Design review of the part built by this model. Coordinates are the model's own, in mm. A direction names the side the tool comes from. Round coordinates to 2 decimals unless told otherwise and drop trailing zeros. Write each loop counter-clockwise with the first axis right and the second up, starting at its lowest first coordinate (ties: lowest second). Pieces come first, ordered by that corner, then holes. Notation, with made-up numbers: M -1.75,-39 L 42.25,-39 A4 cw 42.25,-32 Z; hole C 16.5,29.25 d6. An arc over 180 degrees is marked long. One line per question, with ' | ' between items. Start each with the question number.
Item 1: Insertion check: pin 1 Ø5 at (x, z) = (99.02, 0) entering from -Y; pin 2 Ø5 at (x, z) = (27.98, 0) entering from +Y; pin 3 Ø8 at (x, y) = (101.5, -17.5) entering from -Z. Each pin has a flat end and moves straight along its axis. Give the tip position at first contact, or say it passes through.
Item 2: Machinability: for faces 1 (the face through (63, -25.4, 5)), 2 (the face through (95.917, -28.531, -0.688)), 3 (the face through (127, 3, 0)), 4 (the face through (57.3, 28.62, -1.38)), 5 (the face through (63, 31.75, -11)), which of the approach directions +Z, -Z, +X, -X, +Y, -Y give a long, thin tool a straight path to every point of the face, cutting with its end or side? Answer none if there is none.
Item 3: Draft analysis for pull direction Z (two halves, no side actions). For faces 6 (the face through (24.955, -28.531, 0.954)), 7 (the face through (58, 26, 25.4)), 8 (the face through (58, 26, -25.4)), state which applies: released by +Z, released by -Z, zero draft, split by the parting line, or undercut.
Item 4: Add section B-B, the plane x = 63.5. State the section outline as (y, z) points (3 decimals), and give its area (3 significant figures).
Item 5: Add section A-A, the plane z = 0. State the section outline as (x, y) points (3 decimals).
Item 6: Add section C-C, the plane y = 10. State the section outline as (x, z) points.
Item 7: For L1, parallel to Y at x = 112, z = 4.5; L2, parallel to X at y = 35.5, z = 10, list the stretches that pass through material, from the lowest coordinate up.
Item 8: Add section D-D, the plane z = -12.5. State the section outline as (x, y) points.
```python
from build123d import *

# Parameters (mm, degrees)
SKETCH1_W               = 50.8
SKETCH1_H               = 63.5
BOSS_EXTRUDE1_DEPTH     = 127
SKETCH2_W               = 6.35
SKETCH2_H               = 50.8
BOSS_EXTRUDE2_DEPTH     = 6.35
CUT_EXTRUDE2_DEPTH      = 136.002851822
CUT_EXTRUDE2_DEPTH_BACK = 136.002851822
SKETCH4_W               = 114.3
SKETCH4_H               = 50.8
CUT_EXTRUDE3_REACH      = 146.244
SKETCH5_R               = 6.35
CUT_EXTRUDE4_REACH      = 146.244
SKETCH6_R               = 3.175


with BuildPart() as part:
    # Sketch1 → Boss-Extrude1 (new body)
    with BuildSketch(Plane(origin=(0, 0, 0), x_dir=(0, 0, -1), z_dir=(1, 0, 0))):
        Rectangle(SKETCH1_W, SKETCH1_H)
    extrude(amount=BOSS_EXTRUDE1_DEPTH)

    # Sketch2 → Boss-Extrude2 (add)
    with BuildSketch(Plane(origin=(0, 31.75, 0), x_dir=(1, 0, 0), z_dir=(0, 1, 0))):
        with Locations((123.825, 0)):
            Rectangle(SKETCH2_W, SKETCH2_H)
        with Locations((3.175, 0)):
            Rectangle(SKETCH2_W, SKETCH2_H)
    extrude(amount=BOSS_EXTRUDE2_DEPTH)

    # Sketch4 → Cut-Extrude2 (cut, two sides: drawn at the far end of the back side and taken through both)
    with BuildSketch(Plane.XY.offset(-CUT_EXTRUDE2_DEPTH_BACK)):
        with Locations((63.5, 0)):
            Rectangle(SKETCH4_W, SKETCH4_H)
    extrude(amount=CUT_EXTRUDE2_DEPTH + CUT_EXTRUDE2_DEPTH_BACK, mode=Mode.SUBTRACT)

    # Sketch5 → Cut-Extrude3 (cut, up to next)
    with BuildSketch(Plane(origin=(0, 31.75, 0), x_dir=(1, 0, 0), z_dir=(0, 1, 0)), mode=Mode.PRIVATE) as cut_extrude3_sk1:
        with Locations(Location((63.5, 0, 0), (0, 0, 270))):
            Circle(SKETCH5_R)
    cut_extrude3_tool1 = extrude(cut_extrude3_sk1.sketch, amount=-CUT_EXTRUDE3_REACH, mode=Mode.PRIVATE) & part.part
    add(cut_extrude3_tool1.solids().sort_by_distance((63.5, 31.75, 0))[0], mode=Mode.SUBTRACT)

    # Sketch6 → Cut-Extrude4 (cut, up to next)
    with BuildSketch(Plane(origin=(0, -25.4, 0), x_dir=(1, 0, 0), z_dir=(0, 1, 0)), mode=Mode.PRIVATE) as cut_extrude4_sk1:
        with Locations(Location((63.5, 0, 0), (0, 0, 180))):
            Circle(SKETCH6_R)
    cut_extrude4_tool1 = extrude(cut_extrude4_sk1.sketch, amount=-CUT_EXTRUDE4_REACH, mode=Mode.PRIVATE) & part.part
    # Sketch6 → Cut-Extrude4 (cut, up to next)
    with BuildSketch(Plane(origin=(0, -25.4, 0), x_dir=(1, 0, 0), z_dir=(0, 1, 0)), mode=Mode.PRIVATE) as cut_extrude4_sk2:
        with Locations(Location((27.983351472, 0, 0), (0, 0, 180))):
            Circle(SKETCH6_R)
    cut_extrude4_tool2 = extrude(cut_extrude4_sk2.sketch, amount=-CUT_EXTRUDE4_REACH, mode=Mode.PRIVATE) & part.part
    # Sketch6 → Cut-Extrude4 (cut, up to next)
    with BuildSketch(Plane(origin=(0, -25.4, 0), x_dir=(1, 0, 0), z_dir=(0, 1, 0)), mode=Mode.PRIVATE) as cut_extrude4_sk3:
        with Locations(Location((99.016648528, 0, 0), (0, 0, 270))):
            Circle(SKETCH6_R)
    cut_extrude4_tool3 = extrude(cut_extrude4_sk3.sketch, amount=-CUT_EXTRUDE4_REACH, mode=Mode.PRIVATE) & part.part
    add(cut_extrude4_tool1.solids().sort_by_distance((63.5, -25.4, 0))[0], mode=Mode.SUBTRACT)
    add(cut_extrude4_tool2.solids().sort_by_distance((27.983351, -25.4, 0))[0], mode=Mode.SUBTRACT)
    add(cut_extrude4_tool3.solids().sort_by_distance((99.016649, -25.4, 0))[0], mode=Mode.SUBTRACT)


solid = part.part
```
Computed values:
1) pin 1: stops at y = 25.4 | pin 2: stops at y = 31.75 | pin 3: passes through
2) face 1: +Z, -Z | face 2: -Y | face 3: +Z, -Z, +X, +Y, -Y | face 4: +Y | face 5: +Z, -Z, +Y
3) face 6: undercut | face 7: released by +Z | face 8: released by -Z
4) outline: M -31.75,-25.4 L -25.4,-25.4 L -25.4,-3.175 L -31.75,-3.175 Z; M -31.75,3.175 L -25.4,3.175 L -25.4,25.4 L -31.75,25.4 Z; M 25.4,-25.4 L 31.75,-25.4 L 31.75,-6.35 L 25.4,-6.35 Z; M 25.4,6.35 L 31.75,6.35 L 31.75,25.4 L 25.4,25.4 Z | area: 524 mm^2
5) outline: M 0,-31.75 L 24.808,-31.75 L 24.808,-25.4 L 6.35,-25.4 L 6.35,25.4 L 57.15,25.4 L 57.15,31.75 L 6.35,31.75 L 6.35,38.1 L 0,38.1 Z; M 31.158,-31.75 L 60.325,-31.75 L 60.325,-25.4 L 31.158,-25.4 Z; M 66.675,-31.75 L 95.842,-31.75 L 95.842,-25.4 L 66.675,-25.4 Z; M 69.85,25.4 L 120.65,25.4 L 120.65,-25.4 L 102.192,-25.4 L 102.192,-31.75 L 127,-31.75 L 127,38.1 L 120.65,38.1 L 120.65,31.75 L 69.85,31.75 Z
6) outline: M 0,-25.4 L 6.35,-25.4 L 6.35,25.4 L 0,25.4 Z; M 120.65,-25.4 L 127,-25.4 L 127,25.4 L 120.65,25.4 Z
7) L1: y = -31.75 to -25.4, 25.4 to 31.75 | L2: x = 0 to 6.35, 120.65 to 127
8) outline: M 0,-31.75 L 127,-31.75 L 127,38.1 L 120.65,38.1 L 120.65,31.75 L 6.35,31.75 L 6.35,38.1 L 0,38.1 Z; hole M 6.35,-25.4 L 120.65,-25.4 L 120.65,25.4 L 6.35,25.4 Z
